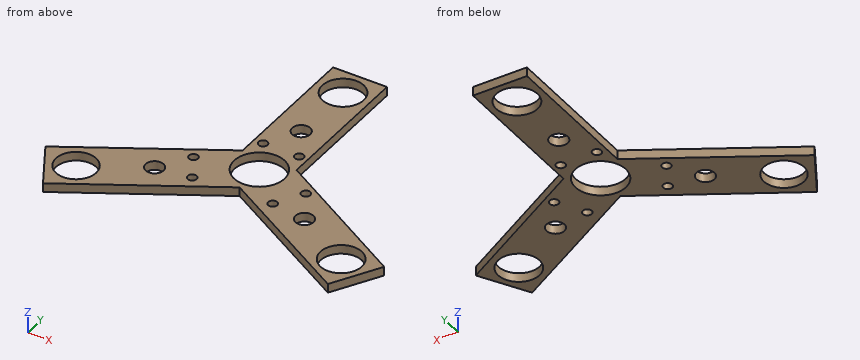
```python
from build123d import *

# Parameters (mm, degrees)
SKETCH1_R           = 28
SKETCH1_R_2         = 23
SKETCH1_R_3         = 22.356889663
SKETCH1_R_4         = 10
BOSS_EXTRUDE5_DEPTH = 10
SKETCH3_R           = 5
CUT_EXTRUDE1_DEPTH  = 261.971545909


with BuildPart() as part:
    # Sketch1 → Boss-Extrude5 (new body)
    with BuildSketch(Plane.XY):
        Polygon((-30, 178), (30, 178), (30, 18), (183.857450853, -71.509132591), (153.857450853, -123.470656818), (-0.295071021, -34.470656818), (-160.583702803, -127.354060192), (-190.583702803, -75.392535965), (-30, 18), align=None)
        Circle(SKETCH1_R, mode=Mode.SUBTRACT)
        with Locations((0, 148)):
            Circle(SKETCH1_R_2, mode=Mode.SUBTRACT)
        with Locations((-149.602940689, -86.373298079)):
            Circle(SKETCH1_R_3, mode=Mode.SUBTRACT)
        with Locations((142.876688739, -82.489894704)):
            Circle(SKETCH1_R_2, mode=Mode.SUBTRACT)
        with Locations((0, 74)):
            Circle(SKETCH1_R_4, mode=Mode.SUBTRACT)
        with Locations((-85.517060809, -49.373298079)):
            Circle(SKETCH1_R_4, mode=Mode.SUBTRACT)
        with Locations((78.790808859, -45.489894704)):
            Circle(SKETCH1_R_4, mode=Mode.SUBTRACT)
    extrude(amount=-BOSS_EXTRUDE5_DEPTH)

    # Sketch3 → Cut-Extrude1 (cut, through all)
    with BuildSketch(Plane.XY):
        with Locations((-63.35415014, -15.760585401)):
            Circle(SKETCH3_R)
        with Locations((-46.739077881, -44.538734725)):
            Circle(SKETCH3_R)
        with Locations((40.201063697, -40.329293976)):
            Circle(SKETCH3_R)
        with Locations((57.836027276, -9.784641068)):
            Circle(SKETCH3_R)
        with Locations((-19.80604921, 38)):
            Circle(SKETCH3_R)
        with Locations((20.434338159, 38)):
            Circle(SKETCH3_R)
    extrude(amount=-CUT_EXTRUDE1_DEPTH, mode=Mode.SUBTRACT)


solid = part.part
```
Input: part model. Units: mm. Frame: model coordinates. Give positions to 0.01 mm unless a question says otherwise; leave off trailing zeros. Loops run counter-clockwise (first coordinate to the right, second up) from the corner with the lowest first, then second, coordinate; pieces in that order, holes last.
1) Line query: L1, parallel to X at y = 34, z = -3.5; L2, parallel to Y at x = 0, z = -5; L3, parallel to X at y = 47, z = -8. Output: solid intervals per line, ascending.
A:
L1: x = -30 to -22.81, -16.81 to 17.43, 23.43 to 30
L2: y = -34.64 to -28, 28 to 64, 84 to 125, 171 to 178
L3: x = -30 to 30
2) Section query C-C on x = -154.5. Return the cut outline in (y, z).
A:
outline: (-123.83, -10) - (-108.19, -10) - (-108.19, 0) - (-123.83, 0) - close; (-64.56, -10) - (-54.41, -10) - (-54.41, 0) - (-64.56, 0) - close
3) Section query D-D on z = -4. Count the separate pieces of the cut face and the enclosed holes in it, and give its area (3 significant figures).
A:
separate pieces: 1
enclosed holes: 13
area: 24,300 mm2
4) Contact query for flat-ended pins moving along their axis: pin 1 (4 mm diameter, centred on x = 59, z = -2, fed in from -Y); pin 2 (11.5 mm diameter, centred on x = 20.43, y = 38, fed in from -Z); pin 3 (1.5 mm diameter, centred on y = -41.5, z = -1.5, fed in from +X); pin 4 (5 mm diameter, centred on y = 125.5, z = -4, fed in from +X). Output: stop coordinate, or through.
A:
pin 1: stops at y = -69.86
pin 2: stops at z = -10
pin 3: stops at x = 133.56
pin 4: stops at x = 30
5) Section query A-A on y = 38. Return the cut outline in (x, z), and give its area (3 significant figures).
A:
outline: (-30, -10) - (-24.81, -10) - (-24.81, 0) - (-30, 0) - close; (-14.81, -10) - (15.43, -10) - (15.43, 0) - (-14.81, 0) - close; (25.43, -10) - (30, -10) - (30, 0) - (25.43, 0) - close
area: 400 mm2
6) Section query B-B on y = 74. Return the cut outline in (x, z), and give its area (3 significant figures).
A:
outline: (-30, -10) - (-10, -10) - (-10, 0) - (-30, 0) - close; (10, -10) - (30, -10) - (30, 0) - (10, 0) - close
area: 400 mm2
